Autodesk Inventor part; units mm, degrees
ref_plane "YZ Plane" through (0, 0, 0) normal (1, 0, 0) x (0, 1, 0)
ref_plane "XZ Plane" through (0, 0, 0) normal (0, 1, 0) x (-1, 0, 0)
ref_plane "XY Plane" through (0, 0, 0) normal (0, 0, 1) x (1, 0, 0)
sketch "Sketch1" plane through (0, 0, 0) normal (0, 1, 0) x (-1, 0, 0)
  line L0 (0, 0) -> (-10, 0)
  line L1 (-10, 0) -> (-10, 20)
  line L2 (-10, 20) -> (0, 20)
  line L3 (0, 20) -> (0, 0)
  dimension "d0" = 10
  dimension "d1" = 20
extrude "Extrusion1" add sketch "Sketch1" along normal blind 5
sketch "Sketch2" plane through (0, 5, 0) normal (0, 1, 0) x (1, 0, 0)
  line L0 (0, 0) -> (0, -20)
  line L1 (0, -15.0001) -> (5, -15.0001)
  line L2 (5, -15.0001) -> (5, -5.0001)
  line L3 (5, -5.0001) -> (0, -5.0001)
  line L4 (0, -5.0001) -> (0, -15.0001)
  dimension "d4" = 5
  dimension "d5" = 10
extrude "Extrusion2" add sketch "Sketch2" along normal blind 8
sketch "Sketch3" plane through (0, 0, 0) normal (-1, 0, 0) x (0, 0, 1)
  circle A0 centre (10.0001, 11.0001) radius 1.5
  point P0 (0, 0)
  dimension "d8" = 3
hole "Hole1" at (0, 11.0001, 10.0001) direction (1, 0, 0) diameter 2.8 end through all
sketch "Sketch4" plane through (0, 0, 0) normal (-1, 0, 0) x (0, 0, 1)
  circle A0 centre (10.0001, 11.0001) radius 1.4
  line L0 (15.0001, 13) -> (5.0001, 13)
  line L1 (8.6001, 11.0001) -> (11.402, 11.0001)
  line L2 (11.402, 11.0001) -> (11.402, 13)
  line L3 (11.402, 13) -> (8.6001, 13)
  line L4 (8.6001, 13) -> (8.6001, 11.0001)
  point P0 (0, 0)
extrude "Extrusion3" cut sketch "Sketch4" against normal blind 9.4625 contours L1 A0 | A0 L4 L0 L2 picked at (10.3893, 11.6381)
sketch "Sketch5" plane through (0, 5, 0) normal (0, 1, 0) x (1, 0, 0)
  point P0 (0, 0)
  point P1 (8.0954, -1.6675)
hole "Hole2" at (8.0954, 5, 1.6675) direction (0, -1, 0) diameter 1 end through all
sketch "Sketch6" plane through (0, 5, 0) normal (0, 1, 0) x (1, 0, 0)
  point P0 (0, 0)
  point P1 (8.1579, -18.3637)
hole "Hole3" at (8.1579, 5, 18.3637) direction (0, -1, 0) diameter 1 end through all
properties part number "laser_uchwyt"
Check sheet for the modelled part. Datum: model origin and axes. Units: mm. A direction names the side the tool comes from. Round coordinates to 2 decimals unless told otherwise and drop trailing zeros. Loops run counter-clockwise (first coordinate to the right, second up) from the corner with the lowest first, then second, coordinate; pieces in that order, holes last. Notation, with made-up numbers: (80.25, 9) - (85.25, 9) arc R23 cw to (85.25, 29) - close; hole circle Ø6 at (25, 10). An arc over 180 degrees is marked (long way). Answer as a JSON object with one key per item and string values. Group by question number.
Q1. Set-up check for faces 1 (the face through (2, 12, 8.6)), 2 (the face through (2, 13, 13)), 3 (the face through (3, 9, 5)), 4 (the face through (7.6, 2.5, 1.6)), 5 (the face through (5, 9, 10)): record each of +Z, -Z, +X, -X, +Y, -Y from which the full face is reachable in a straight line by a thin tool's end or side.
Q2. Mould release check, pull along Z, two halves, no side actions. Record for faces 6 (the face through (2, 12, 11.402)), 7 (the face through (2, 9, 15)), 8 (the face through (7.736, 2.465, 18.632)), 9 (the face through (5, 0, 10)): released by +Z, released by -Z, zero draft, split by the parting line, or undercut.
Q3. Sectioned sample at D-D, the plane y = 10.25. Enter the section's corners in (x, z).
Q4. Gauge pin test, flat ends, axial feed: P1, Ø1, axis at x = 8, y = 6.5, coming from the +Z side; P2, Ø2, axis at x = 7, z = 17, coming from the +Y side; P3, Ø5.5, axis at x = 1.5, y = 9.5, coming from the -Z side; P4, Ø2.5, axis at x = 2.5, y = 7.5, coming from the +Z side. Record the tip position at first contact, or that the pin passes through.
Q5. Sectioned sample at A-A, the plane y = 12. Enter the section's corners in (x, z).
Q6. Sectioned sample at C-C, the plane z = 13. Enter the section's corners in (x, y).
Q7. Sectioned sample at B-B, the plane x = 3.75. Enter the section's corners in (y, z), plus the area to 3 significant figures.
Q8. Scan lines: line 1 along X through (y, z) = (8, 13.5); line 2 along Z through (x, y) = (8.25, 3.75). Record each from-to range of solid material in increasing order. Write a range as [from, to].
Solution:
{
 "1": {"face 1": "+X, -X, +Y", "face 2": "+Z, -Z, +X, -X, +Y", "face 3": "-Z, +X, -X, +Y", "face 4": "+Y, -Y", "face 5": "+Z, -Z, +X, +Y"},
 "2": {"face 6": "undercut", "face 7": "released by +Z", "face 8": "undercut", "face 9": "zero draft"},
 "3": {"outline": "(0, 5) - (5, 5) - (5, 8.82) - (0, 8.82) - close; (0, 11.18) - (5, 11.18) - (5, 15) - (0, 15) - close"},
 "4": {"P1": "passes through", "P2": "stops at y = 5", "P3": "stops at z = 5", "P4": "stops at z = 15"},
 "5": {"outline": "(0, 5) - (5, 5) - (5, 8.6) - (0, 8.6) - close; (0, 11.4) - (5, 11.4) - (5, 15) - (0, 15) - close"},
 "6": {"outline": "(0, 0) - (10, 0) - (10, 5) - (5, 5) - (5, 13) - (0, 13) - close"},
 "7": {"outline": "(0, 0) - (5, 0) - (5, 5) - (13, 5) - (13, 8.6) - (11, 8.6) arc R1.4 cw to (11, 11.4) - (13, 11.4) - (13, 15) - (5, 15) - (5, 20) - (0, 20) - close", "area": "171 mm²"},
 "8": {"line 1": "x = [0, 5]", "line 2": "z = [0, 1.19], [2.14, 17.87], [18.86, 20]"}
}
